Can you work these out from the model? Positions are in its coordinate system, mm. Give positions to 0.01 mm unless a question says otherwise; leave off trailing zeros. Loops run counter-clockwise (first coordinate to the right, second up) from the corner with the lowest first, then second, coordinate; pieces in that order, holes last. Notation, with made-up numbers: (-24.75, 7.25) - (21.25, 7.25) arc R28 cw to (21.25, 26.25) - close; hole circle Ø5 at (76, -29.75). An arc over 180 degrees is marked (long way). Write item = value, one per line.
from build123d import *

# Parameters (mm, degrees)
SKETCH1_R           = 3.2639
SKETCH1_R_2         = 14.2875
SKETCH1_R_3         = 2.4892
BOSS_EXTRUDE1_DEPTH = 4.7625


with BuildPart() as part:
    # Sketch1 → Boss-Extrude1 (new body)
    with BuildSketch(Plane.XY):
        Polygon((76.2, 0), (76.2, 25.4), (50.8, 76.2), (25.4, 76.2), (0, 25.4), (-76.2, 25.4), (-76.2, 0), (-76.2, -215.9), (-76.2, -228.6), (0, -228.6), (0, -203.2), (38.1, -203.2), (88.9, -203.2), (88.9, -165.1), (76.2, -165.1), align=None)
        with Locations(Location((-38.1, 12.7, 0), (0, 0, 180))):
            Circle(SKETCH1_R, mode=Mode.SUBTRACT)
        with Locations(Location((-12.7, 12.7, 0), (0, 0, 180))):
            Circle(SKETCH1_R, mode=Mode.SUBTRACT)
        with Locations(Location((-63.5, 12.7, 0), (0, 0, 180))):
            Circle(SKETCH1_R, mode=Mode.SUBTRACT)
        with Locations(Location((12.7, 12.7, 0), (0, 0, 180))):
            Circle(SKETCH1_R, mode=Mode.SUBTRACT)
        with Locations(Location((38.1, 12.7, 0), (0, 0, 180))):
            Circle(SKETCH1_R, mode=Mode.SUBTRACT)
        with Locations(Location((38.1, 50.8, 0), (0, 0, 180))):
            Circle(SKETCH1_R_2, mode=Mode.SUBTRACT)
        with Locations(Location((63.5, 12.7, 0), (0, 0, 180))):
            Circle(SKETCH1_R, mode=Mode.SUBTRACT)
        with Locations(Location((38.1, -184.15, 0), (0, 0, 180))):
            Circle(SKETCH1_R_2, mode=Mode.SUBTRACT)
        with Locations(Location((38.1, -165.1, 0), (0, 0, 180))):
            Circle(SKETCH1_R_3, mode=Mode.SUBTRACT)
        with Locations(Location((-12.7, -215.9, 0), (0, 0, 180))):
            Circle(SKETCH1_R, mode=Mode.SUBTRACT)
        with Locations(Location((-38.1, -215.9, 0), (0, 0, 180))):
            Circle(SKETCH1_R, mode=Mode.SUBTRACT)
        with Locations(Location((-63.5, -215.9, 0), (0, 0, 180))):
            Circle(SKETCH1_R, mode=Mode.SUBTRACT)
        with Locations(Location((38.1, 69.85, 0), (0, 0, 180))):
            Circle(SKETCH1_R_3, mode=Mode.SUBTRACT)
        with Locations(Location((82.55, -184.15, 0), (0, 0, 180))):
            Circle(SKETCH1_R, mode=Mode.SUBTRACT)
        with Locations(Location((-6.35, -184.15, 0), (0, 0, 180))):
            Circle(SKETCH1_R, mode=Mode.SUBTRACT)
    extrude(amount=BOSS_EXTRUDE1_DEPTH)


solid = part.part
Q1. Imagine slicing it at D-D, the plane x = -12.7. Write out the boundary of the cut face in (y, z), then the cut area to 3 significant figures.
Output:
outline = (-228.6, 0) - (-219.16, 0) - (-219.16, 4.76) - (-228.6, 4.76) - close; (-212.64, 0) - (9.44, 0) - (9.44, 4.76) - (-212.64, 4.76) - close; (15.96, 0) - (25.4, 0) - (25.4, 4.76) - (15.96, 4.76) - close
area = 1,150 mm2
Q2. Imagine slicing it at B-B, the plane z = 2.9. Give the number of separate pieces and of enclosed holes in the cut face, then the cut area to 3 significant figures.
Output:
separate_pieces = 1
enclosed_holes = 15
area = 38,100 mm2
Q3. I need wall thicknesses on L1, parallel to Y at x = 38.5, z = 4.3; L2, parallel to Y at x = 38.1, z = 2.4; L3, parallel to Y at x = -38.1, z = 2.2. Which ranges of each line are inside material? Lowest first, please.
Output:
L1 = -203.2 to -198.43, -169.87 to -167.56, -162.64 to 9.46, 15.94 to 36.52, 65.08 to 67.39, 72.31 to 76.2
L2 = -203.2 to -198.44, -169.86 to -167.59, -162.61 to 9.44, 15.96 to 36.51, 65.09 to 67.36, 72.34 to 76.2
L3 = -228.6 to -219.16, -212.64 to 9.44, 15.96 to 25.4
Q4. Imagine slicing it at A-A, the plane x = 12.7. Write out the boundary of the cut face in (y, z).
Output:
outline = (-203.2, 0) - (9.44, 0) - (9.44, 4.76) - (-203.2, 4.76) - close; (15.96, 0) - (50.8, 0) - (50.8, 4.76) - (15.96, 4.76) - close
Q5. Imagine slicing it at C-C, the plane y = 50.8. Write out the boundary of the cut face in (x, z).
Output:
outline = (12.7, 0) - (23.81, 0) - (23.81, 4.76) - (12.7, 4.76) - close; (52.39, 0) - (63.5, 0) - (63.5, 4.76) - (52.39, 4.76) - close
Q6. For pin 1 (2.5 mm diameter, centred on y = -218.5, z = 3, fed in from +X); pin 2 (1.5 mm diameter, centred on x = 54, z = 0.5, fed in from -Y); pin 3 (2.5 mm diameter, centred on x = -52, z = 1.5, fed in from +Y), each with a flat end and sliding along its axis, tell me the tip position at first contact or that it passes through.
Output:
pin_1 = 0
pin_2 = -203.2
pin_3 = 25.4
Q7. We'd pull the mould along X, two halves only. Please class faces 1 (the flat face through (63.7, 50.4, 2.3)), 2 (the cylindrical face through (61.745, 9.948, 2.348)), 3 (the flat face through (12.9, 51.2, 2.3)), 4 (the flat face through (5, -74, 4.762)): released by +X, released by -X, zero draft, split by the parting line, or undercut.
Output:
face_1 = released by +X
face_2 = undercut
face_3 = released by -X
face_4 = zero draft
